Build history of the part. All positions in model axes, mm. A direction names the side the tool comes from. Coordinates: 2 decimals unless noted, no trailing zeros. Write each loop counter-clockwise with the first axis right and the second up, starting at its lowest first coordinate (ties: lowest second). Pieces come first, ordered by that corner, then holes.
from build123d import *

# Parameters (mm, degrees)
SKETCH1_W           = 54.5
SKETCH1_H           = 34.5
BOSS_EXTRUDE1_DEPTH = 1.5
SKETCH6_W           = 5
SKETCH6_H           = 14.5
CUT_EXTRUDE1_DEPTH  = 2
SKETCH9_W           = 5
SKETCH9_H           = 14.5
CUT_EXTRUDE2_DEPTH  = 2
SKETCH27_W          = 1.5
SKETCH27_H          = 10
CUT_EXTRUDE3_DEPTH  = 2
SKETCH28_W          = 1.5
SKETCH28_H          = 10
CUT_EXTRUDE4_DEPTH  = 2
SKETCH29_W          = 1.5
SKETCH29_H          = 10
CUT_EXTRUDE5_DEPTH  = 2
SKETCH30_W          = 1.5
SKETCH30_H          = 10
CUT_EXTRUDE6_DEPTH  = 2
SKETCH31_W          = 1.5
SKETCH31_H          = 10
CUT_EXTRUDE7_DEPTH  = 2
SKETCH32_W          = 1.5
SKETCH32_H          = 10
CUT_EXTRUDE8_DEPTH  = 2
SKETCH33_W          = 1.5
SKETCH33_H          = 10
CUT_EXTRUDE9_DEPTH  = 2


with BuildPart() as part:
    # Sketch1 → Boss-Extrude1 (new body)
    with BuildSketch(Plane(origin=(0, 0, 0), x_dir=(1, 0, 0), z_dir=(0, 1, 0))):
        Rectangle(SKETCH1_W, SKETCH1_H)
    extrude(amount=BOSS_EXTRUDE1_DEPTH)

    # Sketch6 → Cut-Extrude1 (cut)
    with BuildSketch(Plane(origin=(0, 1.5, 0), x_dir=(1, 0, 0), z_dir=(0, 1, 0))):
        with Locations((-12.75, 6)):
            Rectangle(SKETCH6_W, SKETCH6_H)
    extrude(amount=-CUT_EXTRUDE1_DEPTH, mode=Mode.SUBTRACT)

    # Sketch9 → Cut-Extrude2 (cut)
    with BuildSketch(Plane(origin=(0, 1.5, 0), x_dir=(1, 0, 0), z_dir=(0, 1, 0))):
        with Locations((12.75, 6)):
            Rectangle(SKETCH9_W, SKETCH9_H)
    extrude(amount=-CUT_EXTRUDE2_DEPTH, mode=Mode.SUBTRACT)

    # Sketch27 → Cut-Extrude3 (cut)
    with BuildSketch(Plane(origin=(0, 1.5, 0), x_dir=(1, 0, 0), z_dir=(0, 1, 0))):
        with Locations((-21, -12.25)):
            Rectangle(SKETCH27_W, SKETCH27_H)
    extrude(amount=-CUT_EXTRUDE3_DEPTH, mode=Mode.SUBTRACT)

    # Sketch28 → Cut-Extrude4 (cut)
    with BuildSketch(Plane(origin=(0, 1.5, 0), x_dir=(1, 0, 0), z_dir=(0, 1, 0))):
        with Locations((-14, -12.25)):
            Rectangle(SKETCH28_W, SKETCH28_H)
    extrude(amount=-CUT_EXTRUDE4_DEPTH, mode=Mode.SUBTRACT)

    # Sketch29 → Cut-Extrude5 (cut)
    with BuildSketch(Plane(origin=(0, 1.5, 0), x_dir=(1, 0, 0), z_dir=(0, 1, 0))):
        with Locations((-7, -12.25)):
            Rectangle(SKETCH29_W, SKETCH29_H)
    extrude(amount=-CUT_EXTRUDE5_DEPTH, mode=Mode.SUBTRACT)

    # Sketch30 → Cut-Extrude6 (cut)
    with BuildSketch(Plane(origin=(0, 1.5, 0), x_dir=(1, 0, 0), z_dir=(0, 1, 0))):
        with Locations((0, -12.25)):
            Rectangle(SKETCH30_W, SKETCH30_H)
    extrude(amount=-CUT_EXTRUDE6_DEPTH, mode=Mode.SUBTRACT)

    # Sketch31 → Cut-Extrude7 (cut)
    with BuildSketch(Plane(origin=(0, 1.5, 0), x_dir=(1, 0, 0), z_dir=(0, 1, 0))):
        with Locations((7, -12.25)):
            Rectangle(SKETCH31_W, SKETCH31_H)
    extrude(amount=-CUT_EXTRUDE7_DEPTH, mode=Mode.SUBTRACT)

    # Sketch32 → Cut-Extrude8 (cut)
    with BuildSketch(Plane(origin=(0, 1.5, 0), x_dir=(1, 0, 0), z_dir=(0, 1, 0))):
        with Locations((14, -12.25)):
            Rectangle(SKETCH32_W, SKETCH32_H)
    extrude(amount=-CUT_EXTRUDE8_DEPTH, mode=Mode.SUBTRACT)

    # Sketch33 → Cut-Extrude9 (cut)
    with BuildSketch(Plane(origin=(0, 1.5, 0), x_dir=(1, 0, 0), z_dir=(0, 1, 0))):
        with Locations((21, -12.25)):
            Rectangle(SKETCH33_W, SKETCH33_H)
    extrude(amount=-CUT_EXTRUDE9_DEPTH, mode=Mode.SUBTRACT)


solid = part.part
(1) Two-plate mould, pull along Z, no slides. Class faces 4 (the flat face through (0, 1, -17.25)), 5 (the flat face through (7.75, 1, 12)), 6 (the flat face through (13, 1, -13.25)): pulls with the +Z half, pulls with the -Z half, needs draft (parallel to the pull), parting line crosses it, or undercut.
(2) Slice it at D-D, the plane x = 14. List the corners of the cut face in (y, z).
(3) Slice it at C-C, the plane y = 0.8. Give the number of separate pieces and of enclosed holes in the cut face, and give its area (3 significant figures).
(4) Probe L1, parallel to X at y = 0.9, z = -11.5; L2, parallel to Z at x = 13.5, y = 1.4; L3, parallel to Z at x = -15, y = 1.1. List the from-to ranges inside material, lowest first.
(5) 3-axis set-ups, long thin cutter, end or side, ignore diameter. For faces 1 (the flat face through (17, 1, 17.25)), 2 (the flat face through (13.25, 1, 12)), 3 (the flat face through (15.25, 1, -6)): which of +Z, -Z, +X, -X, +Y, -Y reach the whole face in a straight line?
(6) Slice it at B-B, the plane x = -11. List the corners of the cut face in (y, z), and give its area (3 significant figures).
(7) Slice it at A-A, the plane z = -0.5. List the corners of the cut face in (x, y).
Results:
1. face 4: pulls with the -Z half
1. face 5: needs draft
1. face 6: undercut
2. outline: (0, -17.25) - (1.5, -17.25) - (1.5, -13.25) - (0, -13.25) - close; (0, 1.25) - (1.5, 1.25) - (1.5, 7.25) - (0, 7.25) - close
3. separate pieces: 1
3. enclosed holes: 2
3. area: 1,630 mm2
4. L1: x = -27.25 to -15.25, -10.25 to 10.25, 15.25 to 27.25
4. L2: z = -17.25 to -13.25, 1.25 to 7.25
4. L3: z = -17.25 to -13.25, 1.25 to 17.25
5. face 1: +Z, +X, -X, +Y, -Y
5. face 2: +Z, +Y, -Y
5. face 3: +Y, -Y
6. outline: (0, -17.25) - (1.5, -17.25) - (1.5, -13.25) - (0, -13.25) - close; (0, 1.25) - (1.5, 1.25) - (1.5, 17.25) - (0, 17.25) - close
6. area: 30.0 mm2
7. outline: (-27.25, 0) - (-15.25, 0) - (-15.25, 1.5) - (-27.25, 1.5) - close; (-10.25, 0) - (10.25, 0) - (10.25, 1.5) - (-10.25, 1.5) - close; (15.25, 0) - (27.25, 0) - (27.25, 1.5) - (15.25, 1.5) - close
